The listing builds one solid part. Answer for the finished solid, in the listing's coordinates (mm). A direction names the side the tool comes from. Round coordinates to 2 decimals unless told otherwise and drop trailing zeros. Write each loop counter-clockwise with the first axis right and the second up, starting at its lowest first coordinate (ties: lowest second). Pieces come first, ordered by that corner, then holes. Notation, with made-up numbers: (63.25, -19) - (89.25, -19) arc R12 ccw to (89.25, -1) - close; hole circle Ø6 at (-4.5, -18). An arc over 180 degrees is marked (long way). Return JSON: item names as keys, results as strings. Group by question number.
(1) Section A-A, the plane x = 0 is taken. Write down the section's boundary in (y, z).
(2) Which of the six approach directions +Z, -Z, +X, -X, +Y, -Y give full straight-line access (tool end or side, diameter ignored) to faces 5 (the cylindrical face through (14.985, 35.042, 0.66)), 6 (the cylindrical face through (-41, 5, 0))?
(3) Section C-C, the plane y = 4.5 is taken. Write down the section's boundary in (x, z).
(4) Determine the mould class of faces 1 (the cylindrical face through (-17.16, 23.07, 0.65)), 2 (the cylindrical face through (30.24, 4.93, -1.52)), 3 (the flat face through (21.8, 4.9, 20.6)), 4 (the flat face through (24.14, 4.93, -17.8)) for opening direction Z: +Z half, -Z half, draft (parallel to the pull), parting line (faces both ways), or undercut.
(5) Find the intervals of material crossed by line 1 along Z through (x, y) = (0, 33.8); line 2 along Y through (x, z) = (-7.5, -8); line 3 along X through (y, z) = (3.5, -5), in increasing order. Write a range as [from, to].
(6) Each of these flat-tipped pins is pushed along its axis until it touches: pin 1 (1.5 mm diameter, centred on x = 26, z = -2, fed in from -Y); pin 2 (2 mm diameter, centred on x = -28.5, y = 7, fed in from +Z); pin 3 (15.5 mm diameter, centred on x = -35, z = 0, fed in from +Y); pin 4 (5 mm diameter, centred on y = 22.5, z = -14.5, fed in from +X). Where does it stop, or does it pass through?
(7) Section D-D, the plane y = 15 is taken. Write down the section's boundary in (x, z).
(8) Section B-B, the plane z = 0 is taken. Write down the section's boundary in (x, y).
Autodesk Fusion 360 part; units mm, degrees
sketch "Sketch1" plane through (0, 0, 0) normal (0, 1, 0) x (1, 0, 0)
  circle A0 centre (0, 0) radius 25
  circle A1 centre (0, 0) radius 15
  circle A2 centre (0, 0) radius 10
  circle A3 centre (-35, 0) radius 6
  circle A4 centre (35, -2.1327) radius 6
  arc A5 (-39.2857, 14.3747) -> (-39.2857, -14.3747) centre (-35, 0) ccw
  arc A6 (38.3954, -16.7434) -> (40.1443, 11.9576) centre (35, -2.1327) ccw
  line L0 (8.5738, 23.4838) -> (40.1443, 11.9576)
  line L1 (5.659, -24.3511) -> (38.3954, -16.7434)
  line L2 (-39.2857, 14.3747) -> (-7.1429, 23.9579)
  line L3 (-7.1429, -23.9579) -> (-39.2857, -14.3747)
  arc A7 (8.5738, 23.4838) -> (-7.1429, 23.9579) centre (0, 0) ccw
  arc A8 (-7.1429, -23.9579) -> (5.659, -24.3511) centre (0, 0) ccw
  dimension "d3" = 50
  dimension "d4" = 30
  dimension "d5" = 20
  dimension "d8" = 12
  dimension "d9" = 12
  dimension "d10" = 35
  dimension "d11" = 35
  dimension "d12" = 30
  dimension "d13" = 30
extrude "Extrude1" add sketch "Sketch1" along normal blind 10 contours A0 A6 L0 L1 | A0 A5 L2 L3 makes body 1 at (-31.6163, 0, 10.1046) makes body 2 at (31.0948, 10, 12.0614)
sketch "Sketch2" plane through (0, 0, 0) normal (0, 1, 0) x (1, 0, 0)
  circle A0 centre (0, 0) radius 25
  circle A1 centre (0, 0) radius 15
  dimension "d16" = 50
  dimension "d17" = 30
extrude "Extrude2" add sketch "Sketch2" along normal blind 38 bodies 1 2
sketch "Sketch3" plane through (0, 0, 0) normal (0, 1, 0) x (1, 0, 0)
  circle A0 centre (0, 0) radius 15
  dimension "d20" = 30
extrude "Extrude3" add sketch "Sketch3" along normal blind 38 bodies 1
sketch "Sketch4" plane through (0, 38, 0) normal (0, 1, 0) x (-1, 0, 0)
  circle A0 centre (0, 0) radius 25
  circle A1 centre (0, 0) radius 15
  circle A2 centre (0, 0) radius 10
  dimension "d23" = 30
  dimension "d24" = 20
extrude "Extrude4" cut sketch "Sketch4" along normal mid plane 12 contours A1 bodies 1
extrude "Extrude5" cut 1 faces at (2.7541, 38, -1.0148) along direction (0, 1, 0) mid plane 76 on bodies 1 bodies 1
sketch "Sketch5" plane through (0, 0, 0) normal (1, 0, 0) x (0, 0, -1)
  circle A0 centre (0, 26) radius 3
  point P0 (0, 38)
  dimension "d29" = 6
  dimension "d30" = 12
extrude "Extrude6" cut sketch "Sketch5" against normal blind 25 bodies 1
sketch "Sketch6" plane through (0, 0, 0) normal (1, 0, 0) x (0, 0, -1)
Working result:
{
 "1": {"outline": "(0, -25) - (38, -25) - (38, -15) - (32, -15) - (32, -10) - (0, -10) - close; (0, 10) - (32, 10) - (32, 15) - (38, 15) - (38, 25) - (0, 25) - close"},
 "2": {"face 5": "+Y", "face 6": "+Y, -Y"},
 "3": {"outline": "(-39.29, -14.37) - (-7.14, -23.96) arc R25 ccw to (8.57, -23.48) - (40.14, -11.96) arc R15 ccw to (38.4, 16.74) - (5.66, 24.35) arc R25 ccw to (-7.14, 23.96) - (-39.29, 14.37) arc R15 ccw to start; hole circle Ø12 at (-35, 0); hole circle Ø20 at (0, 0); hole circle Ø12 at (35, 2.13)"},
 "4": {"face 1": "undercut", "face 2": "undercut", "face 3": "+Z half", "face 4": "-Z half"},
 "5": {"line 1": "z = [-25, -15], [15, 25]", "line 2": "y = [0, 32]", "line 3": "x = [-49.14, -38.32], [-31.68, -8.66], [8.66, 48.2]"},
 "6": {"pin 1": "stops at y = 0", "pin 2": "stops at z = 17.89", "pin 3": "stops at y = 10", "pin 4": "stops at x = 21.93"},
 "7": {"outline": "circle Ø50 at (0, 0); hole circle Ø20 at (0, 0)"},
 "8": {"outline": "(-50, 0) - (-41, 0) - (-41, 10) - (-50, 10) - close; (-29, 0) - (-10, 0) - (-10, 23) - (-25, 23) - (-25, 10) - (-29, 10) - close; (-25, 29) - (-10, 29) - (-10, 32) - (-15, 32) - (-15, 38) - (-25, 38) - close; (10, 0) - (29.39, 0) - (29.39, 10) - (25, 10) - (25, 38) - (15, 38) - (15, 32) - (10, 32) - close; (40.61, 0) - (49.85, 0) - (49.85, 10) - (40.61, 10) - close"}
}
